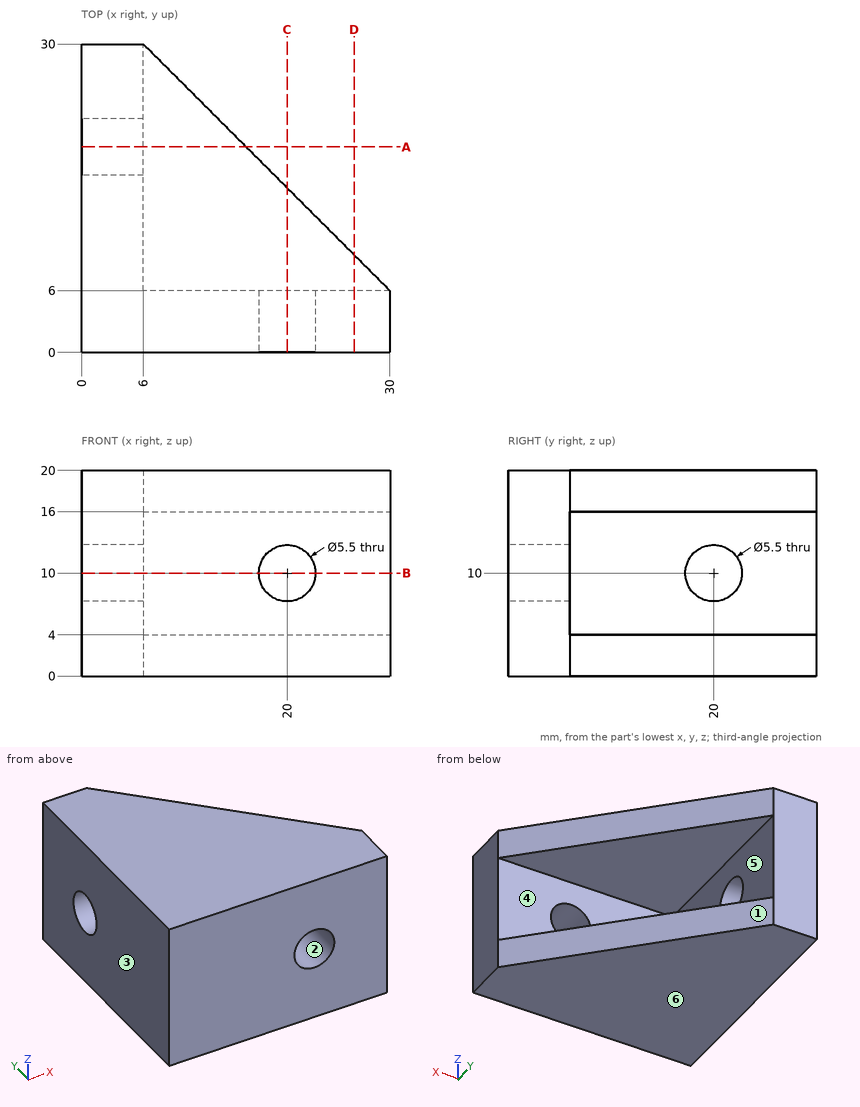
Could you check a few things on this drawing? It's one solid part, dimensions in mm from its lowest x, y, z. A direction names the side the tool comes from. Coordinates: 2 decimals unless noted, no trailing zeros. Order: outer loops, then holes, each group sorted by start corner. A loop starts at its lowest first (then second) coordinate and runs counter-clockwise, first axis right, second up. Notation, with made-up numbers: M 75,-19 L 84,-19 A22 ccw 84,13 Z; hole C -15,-31.5 d3. An arc over 180 degrees is marked long. Use a Markdown table: item, result. Add a question column.
Q1. We'd pull the mould along X, two halves only. Please class the marked faces 1, 2, 3 and 4: pulls with the +X half, pulls with the -X half, needs draft (parallel to the pull), parting line crosses it, or undercut.
Q2. I want a section at B-B on z = 10. List the corners of the cut face in (x, y) for me.
Q3. I want a section at D-D on x = 26.5. List the corners of the cut face in (y, z) for me, then the cut area to 3 significant figures.
Q4. Which directions (+Z, -Z, +X, -X, +Y, -Y) give clear straight access to the entire face, cutting with the end or side of a thin tool? Please do the marked faces 5 and 6.
Q5. I'm going to push flat-ended pins straight in: pin 1 (7 mm diameter, centred on x = 20, z = 10, fed in from +Y); pin 2 (7 mm diameter, centred on y = 20, z = 10, fed in from +X); pin 3 (1.5 mm diameter, centred on x = 24, z = 2, fed in from +Y). Where does each tip first touch, or does it pass through?
Q6. I want a section at A-A on y = 20. List the corners of the cut face in (x, z) for me, then the cut area to 3 significant figures.
Q7. If I drill on L1, parallel to Y at x = 2.8, z = 10; L2, parallel to Z at x = 18, y = 10.5; L3, parallel to X at y = 16, z = 9, over which ranges is the centre line in solid material (lowest first)?
Checked values:
| question | item | result |
|---|---|---|
| 1 | face 1 | pulls with the +X half |
| 1 | face 2 | undercut |
| 1 | face 3 | pulls with the -X half |
| 1 | face 4 | needs draft |
| 2 | outline | M 0,0 L 17.25,0 L 17.25,6 L 6,6 L 6,17.25 L 0,17.25 Z; M 0,22.75 L 6,22.75 L 6,30 L 0,30 Z; M 22.75,0 L 30,0 L 30,6 L 22.75,6 Z |
| 3 | outline | M 0,0 L 9.5,0 L 9.5,4 L 6,4 L 6,16 L 9.5,16 L 9.5,20 L 0,20 Z |
| 3 | area | 148 mm² |
| 4 | face 5 | +X, +Y |
| 4 | face 6 | -Z, +X, -X, +Y, -Y |
| 5 | pin 1 | y = 6 |
| 5 | pin 2 | x = 6 |
| 5 | pin 3 | y = 12.75 |
| 6 | outline | M 0,0 L 16,0 L 16,4 L 6,4 L 6,7.25 L 0,7.25 Z; M 0,12.75 L 6,12.75 L 6,16 L 16,16 L 16,20 L 0,20 Z |
| 6 | area | 167 mm² |
| 7 | L1 | 0 to 17.25, 22.75 to 30 |
| 7 | L2 | 0 to 4, 16 to 20 |
| 7 | L3 | 0 to 6 |
